```python
from build123d import *

# Parameters (mm, degrees)
SWEEP1_PROFILE_R = 0.6


with BuildPart() as part:
    # Sweep1: sweep along a path in Sketch1
    with BuildLine(Plane.XY) as sweep1_path:
        Line((0, 0), (0, 10))
        ThreePointArc((0, 10), (2.928932188, 17.071067812), (10, 20))
        Line((10, 20), (170, 20))
        ThreePointArc((170, 20), (177.071067812, 22.928932188), (180, 30))
        Line((180, 30), (180, 40))
    # Sweep1 profile (on start of the path) → Sweep1 (sweep)
    with BuildSketch(Plane.ZX):
        Circle(SWEEP1_PROFILE_R)
    sweep(path=sweep1_path.line)


solid = part.part
```
Work out the finished part from the listing and answer in its coordinate system (mm). Give positions to 0.01 mm unless a question says otherwise; leave off trailing zeros. Loops run counter-clockwise (first coordinate to the right, second up) from the corner with the lowest first, then second, coordinate; pieces in that order, holes last. Notation, with made-up numbers: (6, 38) -> (39, 38) arc R21 ccw to (39, 74) -> close; hole circle Ø7 at (12.25, -36). An arc over 180 degrees is marked (long way). Put each result on its own line as item: value. Start each with the question number.
Item 1: The part is cut by section A-A (z = 0). Give the vertices of the cut face in (x, y), then the cut area to 3 significant figures.
Item 2: The part is cut by section B-B (x = 23). Give the vertices of the cut face in (y, z), then the cut area to 3 significant figures.
Item 3: Find the intervals of material crossed by L1, parallel to X at y = 29.5, z = 0; L2, parallel to Y at x = 9.5, z = 0.05; L3, parallel to Y at x = 74.5, z = 0.4, in increasing order. Write a range as [from, to].
Answers below:
1. outline: (-0.6, 0) -> (0.6, 0) -> (0.6, 10) arc R9.4 cw to (10, 19.4) -> (170, 19.4) arc R10.6 ccw to (180.6, 30) -> (180.6, 40) -> (179.4, 40) -> (179.4, 30) arc R9.4 cw to (170, 20.6) -> (10, 20.6) arc R10.6 ccw to (-0.6, 10) -> close
1. area: 254 mm2
2. outline: circle Ø1.2 at (20, 0)
2. area: 1.13 mm2
3. L1: [179.39, 180.59]
3. L2: [19.39, 20.59]
3. L3: [19.55, 20.45]
